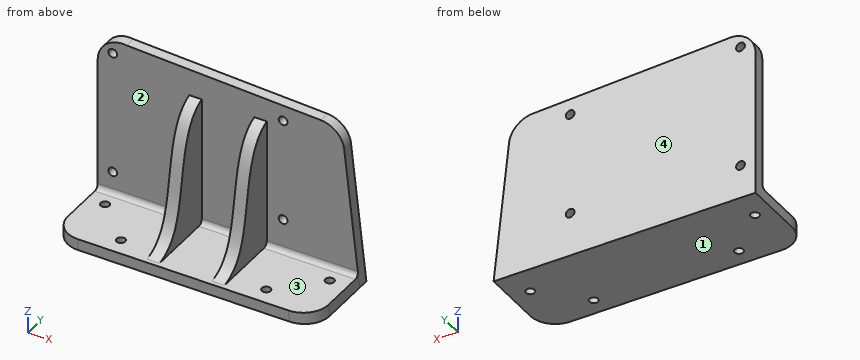
from build123d import *

# Parameters (mm, degrees)
SKETCH2_W           = 132.54933421
SKETCH2_H           = 96.472398488
BOSS_EXTRUDE1_DEPTH = 4.5
CUT_EXTRUDE1_REACH  = 84.093
SKETCH3_R           = 1.75
CUT_EXTRUDE2_REACH  = 84.093
SKETCH4_W           = 132.54933421
SKETCH4_H           = 96.472398488
FILLET1_R           = 10
BOSS_EXTRUDE2_DEPTH = 30
FILLET2_R           = 10
CUT_EXTRUDE3_REACH  = 91.266
SKETCH6_R           = 1.75
RIB1_START          = -2.5
RIB1_DEPTH          = 5
RIB2_START          = -2.5
RIB2_DEPTH          = 5
FILLET3_R           = 2


with BuildPart() as part:
    # Sketch2 → Boss-Extrude1 (new body)
    with BuildSketch(Plane(origin=(0, 0, 0), x_dir=(1, 0, 0), z_dir=(0, 1, 0))):
        Rectangle(SKETCH2_W, SKETCH2_H)
    extrude(amount=BOSS_EXTRUDE1_DEPTH)

    # Sketch3 → Cut-Extrude1 (cut, up to next)
    with BuildSketch(Plane(origin=(0, 4.5, 0), x_dir=(1, 0, 0), z_dir=(0, 1, 0)), mode=Mode.PRIVATE) as cut_extrude1_sk1:
        with Locations(Location((-43.735552551, 28.375291395, 0), (0, 0, 270))):
            Circle(SKETCH3_R)
    cut_extrude1_tool1 = extrude(cut_extrude1_sk1.sketch, amount=-CUT_EXTRUDE1_REACH, mode=Mode.PRIVATE) & part.part
    # Sketch3 → Cut-Extrude1 (cut, up to next)
    with BuildSketch(Plane(origin=(0, 4.5, 0), x_dir=(1, 0, 0), z_dir=(0, 1, 0)), mode=Mode.PRIVATE) as cut_extrude1_sk2:
        with Locations(Location((-43.735552551, -20.948558002, 0), (0, 0, 270))):
            Circle(SKETCH3_R)
    cut_extrude1_tool2 = extrude(cut_extrude1_sk2.sketch, amount=-CUT_EXTRUDE1_REACH, mode=Mode.PRIVATE) & part.part
    # Sketch3 → Cut-Extrude1 (cut, up to next)
    with BuildSketch(Plane(origin=(0, 4.5, 0), x_dir=(1, 0, 0), z_dir=(0, 1, 0)), mode=Mode.PRIVATE) as cut_extrude1_sk3:
        with Locations(Location((24.372618491, -16.816583266, 0), (0, 0, 270))):
            Circle(SKETCH3_R)
    cut_extrude1_tool3 = extrude(cut_extrude1_sk3.sketch, amount=-CUT_EXTRUDE1_REACH, mode=Mode.PRIVATE) & part.part
    # Sketch3 → Cut-Extrude1 (cut, up to next)
    with BuildSketch(Plane(origin=(0, 4.5, 0), x_dir=(1, 0, 0), z_dir=(0, 1, 0)), mode=Mode.PRIVATE) as cut_extrude1_sk4:
        with Locations(Location((24.372618491, 24.243316659, 0), (0, 0, 270))):
            Circle(SKETCH3_R)
    cut_extrude1_tool4 = extrude(cut_extrude1_sk4.sketch, amount=-CUT_EXTRUDE1_REACH, mode=Mode.PRIVATE) & part.part
    add(cut_extrude1_tool1.solids().sort_by_distance((-43.735553, 4.5, -28.375291))[0], mode=Mode.SUBTRACT)
    add(cut_extrude1_tool2.solids().sort_by_distance((-43.735553, 4.5, 20.948558))[0], mode=Mode.SUBTRACT)
    add(cut_extrude1_tool3.solids().sort_by_distance((24.372618, 4.5, 16.816583))[0], mode=Mode.SUBTRACT)
    add(cut_extrude1_tool4.solids().sort_by_distance((24.372618, 4.5, -24.243317))[0], mode=Mode.SUBTRACT)

    # Sketch4 → Cut-Extrude2 (cut, up to next)
    with BuildSketch(Plane(origin=(0, 4.5, 0), x_dir=(1, 0, 0), z_dir=(0, 1, 0)), mode=Mode.PRIVATE) as cut_extrude2_sk1:
        Rectangle(SKETCH4_W, SKETCH4_H)
        with BuildLine():
            Line((-49.755679651, -16.286633303), (-49.755679651, 41.820488279))
            Line((-49.755679651, 41.820488279), (54.978186069, 41.820488279))
            Line((54.978186069, 41.820488279), (47.882417092, -22.041432557))
            Line((47.882417092, -22.041432557), (-38.186956222, -26.162822184))
            ThreePointArc((-38.186956222, -26.162822184), (-46.248474339, -23.892132442), (-49.755679651, -16.286633303))
        make_face(mode=Mode.SUBTRACT)
    cut_extrude2_tool1 = extrude(cut_extrude2_sk1.sketch, amount=-CUT_EXTRUDE2_REACH, mode=Mode.PRIVATE) & part.part
    add(cut_extrude2_tool1.solids().sort_by_distance((-64.635269, 4.5, 0))[0], mode=Mode.SUBTRACT)

    # Fillet1
    fillet1_edges = [part.edges().sort_by_distance(p)[0] for p in [
        (47.882417092, 2.25, 22.041432557),
    ]]
    fillet(fillet1_edges, radius=FILLET1_R)

    # Sketch5 → Boss-Extrude2 (add)
    with BuildSketch(Plane.XZ):
        Polygon((-49.755679651, -37.320488279), (-49.755679651, -41.820488279), (54.978186069, -41.820488279), (54.478186069, -37.320488279), align=None)
    extrude(amount=BOSS_EXTRUDE2_DEPTH)

    # Fillet2
    fillet2_edges = [part.edges().sort_by_distance(p)[0] for p in [
        (-49.755679651, -30, -39.570488279),
        (54.728186069, -30, -39.570488279),
    ]]
    fillet(fillet2_edges, radius=FILLET2_R)

    # Sketch6 → Cut-Extrude3 (cut, up to next)
    with BuildSketch(Plane.XY.offset(-37.320488279), mode=Mode.PRIVATE) as cut_extrude3_sk1:
        with Locations((-42.5984485, -7.071067812)):
            Circle(SKETCH6_R)
    cut_extrude3_tool1 = extrude(cut_extrude3_sk1.sketch, amount=-CUT_EXTRUDE3_REACH, mode=Mode.PRIVATE) & part.part
    # Sketch6 → Cut-Extrude3 (cut, up to next)
    with BuildSketch(Plane.XY.offset(-37.320488279), mode=Mode.PRIVATE) as cut_extrude3_sk2:
        with Locations((-26.740584124, -22.928932188)):
            Circle(SKETCH6_R)
    cut_extrude3_tool2 = extrude(cut_extrude3_sk2.sketch, amount=-CUT_EXTRUDE3_REACH, mode=Mode.PRIVATE) & part.part
    # Sketch6 → Cut-Extrude3 (cut, up to next)
    with BuildSketch(Plane.XY.offset(-37.320488279), mode=Mode.PRIVATE) as cut_extrude3_sk3:
        with Locations(Location((31.415995213, -22.988580525, 0), (0, 0, 180))):
            Circle(SKETCH6_R)
    cut_extrude3_tool3 = extrude(cut_extrude3_sk3.sketch, amount=-CUT_EXTRUDE3_REACH, mode=Mode.PRIVATE) & part.part
    # Sketch6 → Cut-Extrude3 (cut, up to next)
    with BuildSketch(Plane.XY.offset(-37.320488279), mode=Mode.PRIVATE) as cut_extrude3_sk4:
        with Locations(Location((47.306355451, -7.163278737, 0), (0, 0, 180))):
            Circle(SKETCH6_R)
    cut_extrude3_tool4 = extrude(cut_extrude3_sk4.sketch, amount=-CUT_EXTRUDE3_REACH, mode=Mode.PRIVATE) & part.part
    add(cut_extrude3_tool1.solids().sort_by_distance((-42.598449, -7.071068, -37.320488))[0], mode=Mode.SUBTRACT)
    add(cut_extrude3_tool2.solids().sort_by_distance((-26.740584, -22.928932, -37.320488))[0], mode=Mode.SUBTRACT)
    add(cut_extrude3_tool3.solids().sort_by_distance((31.415995, -22.988581, -37.320488))[0], mode=Mode.SUBTRACT)
    add(cut_extrude3_tool4.solids().sort_by_distance((47.306355, -7.163279, -37.320488))[0], mode=Mode.SUBTRACT)

    # Rib1: read off the stored shape, not the designer's step
    # Rib1 outline → Rib1 (add)
    with BuildSketch(Plane(origin=(-10.638742437, 0.010911634, 0), x_dir=(0.001025650165390613, 0.9999994740207309, 0), z_dir=(0.9999994740207307, -0.0010256501653906128, 0)).offset(RIB1_START)):
        with BuildLine():
            Line((-0.008347513, -37.320488279), (-0.008347513, 14.309096835))
            Line((-0.008347513, 14.309096835), (-0.051031921, 14.294776029))
            add(Edge.make_bspline(
                [(-28.165704325, -37.320488279), (-16.507311445, -35.163666341), (-13.858586231, -11.343701008), (-8.750641214, 11.37601897), (-0.051031921, 14.294776029)],
                knots=[0, 0, 0, 0, 0.549950709, 1, 1, 1, 1], degree=3))
            Line((-28.165704325, -37.320488279), (-0.008347513, -37.320488279))
        make_face()
    extrude(amount=RIB1_DEPTH)

    # Rib2: read off the stored shape, not the designer's step
    # Rib2 outline → Rib2 (add)
    with BuildSketch(Plane(origin=(15.361243887, -0.015755271, 0), x_dir=(0.001025650165390613, 0.9999994740207309, 0), z_dir=(0.9999994740207307, -0.0010256501653906128, 0)).offset(RIB2_START)):
        with BuildLine():
            Line((0.018319406, -37.320488279), (0.018319406, 14.318043703))
            Line((0.018319406, 14.318043703), (-0.051031921, 14.294776029))
            add(Edge.make_bspline(
                [(-28.165704325, -37.320488279), (-16.507311445, -35.163666341), (-13.858586231, -11.343701008), (-8.750641214, 11.37601897), (-0.051031921, 14.294776029)],
                knots=[0, 0, 0, 0, 0.549950709, 1, 1, 1, 1], degree=3))
            Line((-28.165704325, -37.320488279), (0.018319406, -37.320488279))
        make_face()
    extrude(amount=RIB2_DEPTH)

    # Fillet3
    fillet3_edges = [part.edges().sort_by_distance(p)[0] for p in [
        (-31.447217297, 0, -37.320488279),
        (2.361253209, 0, -37.320488279),
        (36.169723715, 0, -37.320488279),
    ]]
    fillet(fillet3_edges, radius=FILLET3_R)


solid = part.part
Input: part model. Units: mm. Frame: model coordinates. Face numbers are marked on the shaded views. A direction names the side the tool comes from. Give positions to 0.01 mm unless a question says otherwise; leave off trailing zeros. Write each loop counter-clockwise with the first axis right and the second up, starting at its lowest first coordinate (ties: lowest second). Pieces come first, ordered by that corner, then holes. Notation, with made-up numbers: M -10,-33.5 L 0,-33.5 A20 cw 0,2.5 Z; hole C 58,36.5 d7. An arc over 180 degrees is marked long. Write item = value, one per line. Start each with the question number.
1) Cut plane C-C on x = 35. Return the cut outline in (y, z), then the cut area to 3 significant figures.
2) First-contact query: pin 1 Ø4 at (x, z) = (24.37, -24.24) entering from -Y; pin 2 Ø2 at (y, z) = (-10.5, -20) entering from +X; pin 3 Ø12 at (x, z) = (-37.5, -31) entering from -Y. Flat tips, straight axial feed; report the tip coordinate or a pass-through.
3) Reachability of the marked faces 1 and 2 from +Z, -Z, +X, -X, +Y, -Y: full face, straight path, thin tool, end or side. Return the list, or none.
4) Draft query along X for the marked faces 3 and 4. Return one class per face: +X half, -X half, draft (parallel to the pull), parting line (faces both ways), or undercut.
5) Material intervals for line 1 along X through (y, z) = (-8, -23); line 2 along Z through (x, y) = (-19, -5); line 3 along Y through (x, z) = (34, 10.5), sorted ascending. Write a range as [from, to].
6) Cut plane A-A on x = 2. Return the cut outline in (y, z).
7) Cut plane B-B on y = 2.5. Return the cut outline in (x, z), then the cut area to 3 significant figures.
Solved:
q1.outline = M -30,-41.82 L 4.5,-41.82 L 4.5,22.66 L 0,22.66 L 0,-35.32 A2 cw -2,-37.32 L -30,-37.32 Z
q1.area = 426 mm2
q2.pin_1 = 0
q2.pin_2 = 17.85
q2.pin_3 = -0.91
q3.face_1 = -Z, +X, -X, +Y, -Y
q3.face_2 = +Z, -Y
q4.face_3 = undercut
q4.face_4 = draft
q5.line_1 = [-13.15, -8.15], [12.85, 17.85]
q5.line_2 = [-41.82, -37.32]
q5.line_3 = [0, 4.5]
q6.outline = M -30,-41.82 L 4.5,-41.82 L 4.5,24.24 L 0,24.24 L 0,-35.32 A2 cw -2,-37.32 L -30,-37.32 Z
q7.outline = M -49.76,-41.82 L 54.98,-41.82 L 48.82,13.57 A10 ccw 39.36,22.45 L -38.19,26.16 A10 ccw -49.76,16.29 Z; hole C -43.74,-28.38 d3.5; hole C -43.74,20.95 d3.5; hole C 24.37,-24.24 d3.5; hole C 24.37,16.82 d3.5
q7.area = 6,610 mm2
